from build123d import *

# Parameters (mm, degrees)
EXTRUDE_1_DEPTH    = 34
HOLE_WIZARD_M8_1_D = 6.8


with BuildPart() as part:
    # 草图1 → 凸台-拉伸1 (new body)
    with BuildSketch(Plane.XY):
        with BuildLine():
            Line((-6.350003001, -5.180792426), (5.989996999, -5.180792426))
            Line((5.989996999, -5.180792426), (10.239996999, -0.930792426))
            Line((10.239996999, -0.930792426), (10.239996999, 2.299207574))
            ThreePointArc((10.239996999, 2.299207574), (10.152129033, 2.511339608), (9.939996999, 2.599207574))
            Line((9.939996999, 2.599207574), (3.819996999, 2.599207574))
            Line((3.819996999, 2.599207574), (3.819996999, 5.789207574))
            ThreePointArc((3.819996999, 5.789207574), (3.732129033, 6.001339608), (3.519996999, 6.089207574))
            Line((3.519996999, 6.089207574), (-3.880003001, 6.089207574))
            ThreePointArc((-3.880003001, 6.089207574), (-4.092135036, 6.001339608), (-4.180003001, 5.789207574))
            Line((-4.180003001, 5.789207574), (-4.180003001, 2.599207574))
            Line((-4.180003001, 2.599207574), (-10.300003001, 2.599207574))
            ThreePointArc((-10.300003001, 2.599207574), (-10.512135036, 2.511339608), (-10.600003001, 2.299207574))
            Line((-10.600003001, 2.299207574), (-10.600003001, -0.930792426))
            Line((-10.600003001, -0.930792426), (-6.350003001, -5.180792426))
        make_face()
    extrude(amount=EXTRUDE_1_DEPTH)

    # M8 螺纹孔1 (through all)
    with Locations(Plane(origin=(0, 6.089207574, 0), x_dir=(-1, 0, 0), z_dir=(0, 1, 0))):
        with Locations((0.180003001, 7), (0.180003001, 27)):
            Hole(HOLE_WIZARD_M8_1_D / 2)


solid = part.part
Work out the finished part from the listing and answer in its coordinate system (mm). A direction names the side the tool comes from. Give positions to 0.01 mm unless a question says otherwise; leave off trailing zeros. Write each loop counter-clockwise with the first axis right and the second up, starting at its lowest first coordinate (ties: lowest second). Pieces come first, ordered by that corner, then holes.
Q1. For a pull along X with two mould halves and no side action, classify faces 1 (the face through (10.24, 1, 17)), 2 (the face through (0, -5.181, 17)), 3 (the face through (-0.92, 0.38, 3.68)) as released by +X, released by -X, zero draft, split by the parting line, or undercut.
Answer:
face 1: released by +X
face 2: zero draft
face 3: undercut
Q2. The part is cut by section A-A on z = 4. Give the vertices of the cut face in (x, y).
Answer:
outline: (-10.6, -0.93) - (-6.35, -5.18) - (-1.78, -5.18) - (-1.78, 6.09) - (-3.88, 6.09) arc R0.3 ccw to (-4.18, 5.79) - (-4.18, 2.6) - (-10.3, 2.6) arc R0.3 ccw to (-10.6, 2.3) - close; (1.42, -5.18) - (5.99, -5.18) - (10.24, -0.93) - (10.24, 2.3) arc R0.3 ccw to (9.94, 2.6) - (3.82, 2.6) - (3.82, 5.79) arc R0.3 ccw to (3.52, 6.09) - (1.42, 6.09) - close
Q3. The part is cut by section D-D on x = 1.75. Give the vertices of the cut face in (y, z).
Answer:
outline: (-5.18, 0) - (6.09, 0) - (6.09, 4.2) - (-5.18, 4.2) - close; (-5.18, 9.8) - (6.09, 9.8) - (6.09, 24.2) - (-5.18, 24.2) - close; (-5.18, 29.8) - (6.09, 29.8) - (6.09, 34) - (-5.18, 34) - close
Q4. A tool of negligible diameter and unlimited length cuts with its end or side. For faces 4 (the face through (0, 6.089, 17)), 5 (the face through (7, 2.599, 17)), 6 (the face through (-7, 2.599, 17)), from which of +Z, -Z, +X, -X, +Y, -Y can it reach the whole face along a straight path? Write none if from no direction.
Answer:
face 4: +Z, -Z, +X, -X, +Y
face 5: +Z, -Z, +X, +Y
face 6: +Z, -Z, -X, +Y
Q5. Given pin 1 (3 mm diameter, centred on x = -8, z = 25.5, fed in from +Y); pin 2 (1 mm diameter, centred on y = 4, z = 12.5, fed in from -X); pin 3 (1 mm diameter, centred on x = -5, y = 3.5, fed in from +Z); pin 4 (1 mm diameter, centred on y = 4, z = 10.5, fed in from +X), each flat-ended and moving along its own axis, determine where each tip first touches the part or whether it passes through.
Answer:
pin 1: stops at y = 2.6
pin 2: stops at x = -4.18
pin 3: passes through
pin 4: stops at x = 3.82
Q6. The part is cut by section B-B on y = -0.25. Give the vertices of the cut face in (x, z), and give its area (3 significant figures).
Answer:
outline: (-10.6, 0) - (10.24, 0) - (10.24, 34) - (-10.6, 34) - close; hole circle Ø6.8 at (-0.18, 7); hole circle Ø6.8 at (-0.18, 27)
area: 636 mm2
Q7. Straight lines are drawn through the part: L1, parallel to Z at x = 2, y = -4.5; L2, parallel to Z at x = -0.25, y = 2; L3, parallel to X at y = 4.25, z = 25. For each, find the intervals that lie inside material, in ascending order.
Answer:
L1: z = 0 to 4.39, 9.61 to 24.39, 29.61 to 34
L2: z = 0 to 3.6, 10.4 to 23.6, 30.4 to 34
L3: x = -4.18 to -2.93, 2.57 to 3.82
Q8. The part is cut by section C-C on z = 12. Give the vertices of the cut face in (x, y).
Answer:
outline: (-10.6, -0.93) - (-6.35, -5.18) - (5.99, -5.18) - (10.24, -0.93) - (10.24, 2.3) arc R0.3 ccw to (9.94, 2.6) - (3.82, 2.6) - (3.82, 5.79) arc R0.3 ccw to (3.52, 6.09) - (-3.88, 6.09) arc R0.3 ccw to (-4.18, 5.79) - (-4.18, 2.6) - (-10.3, 2.6) arc R0.3 ccw to (-10.6, 2.3) - close
